```python
from build123d import *

# Parameters (mm, degrees)
SKETCH2_W = 2
SKETCH2_H = 3


with BuildPart() as part:
    # Sweep1: sweep along a path in Sketch1
    with BuildLine(Plane(origin=(0, 0, 0), x_dir=(1, 0, 0), z_dir=(0, 1, 0))) as sweep1_path:
        Line((5.441400564, 4.563847428), (1.294095226, 3.452580312))
        ThreePointArc((1.294095226, 3.452580312), (0, 3.282209443), (-1.294095226, 3.452580312))
        Line((-1.294095226, 3.452580312), (-4.053171996, 4.191872704))
        ThreePointArc((-4.053171996, 4.191872704), (-5.890289303, 3.131212533), (-4.829629131, 1.294095226))
        Line((-4.829629131, 1.294095226), (4.829629131, -1.294095226))
        ThreePointArc((4.829629131, -1.294095226), (5.890289303, -3.131212533), (4.053171996, -4.191872704))
        Line((4.053171996, -4.191872704), (1.294095226, -3.452580312))
        ThreePointArc((1.294095226, -3.452580312), (0, -3.282209443), (-1.294095226, -3.452580312))
        Line((-1.294095226, -3.452580312), (-5.441400564, -4.563847428))
    # Sketch2 → Sweep1 (sweep)
    with BuildSketch(Plane(origin=(-5.441400564, 0, 4.563847428), x_dir=(0.2588190451025149, 0, 0.96592582628907), z_dir=(-0.96592582628907, 0, 0.2588190451025149))):
        Rectangle(SKETCH2_W, SKETCH2_H)
    sweep(path=sweep1_path.line)


solid = part.part
```
Can you work these out from the model? Positions are in its coordinate system, mm. A direction names the side the tool comes from. Round coordinates to 2 decimals unless told otherwise and drop trailing zeros. Loops run counter-clockwise (first coordinate to the right, second up) from the corner with the lowest first, then second, coordinate; pieces in that order, holes last. Notation, with made-up numbers: M 3.25,49 L 29.25,49 A25 cw 29.25,81 Z; hole C -15.75,-10.5 d2. An arc over 180 degrees is marked long. Answer as a JSON object with one key per item and string values. Group by question number.
Q1. Imagine slicing it at B-B, the plane x = 0.25. Please give me the cut outline in (y, z), then the cut area to 3 significant figures.
Q2. Imagine slicing it at C-C, the plane z = 3. Please give me the cut outline in (x, y).
Q3. Please list where these lines run through material, in increasing order: L1, parallel to Z at x = -0.5, y = 0.65; L2, parallel to Z at x = 1.75, y = 1.3; L3, parallel to Z at x = 5, y = -0.35.
Q4. Imagine slicing it at D-D, the plane x = 2. Please give me the cut outline in (y, z), then the cut area to 3 significant figures.
Q5. We'd pull the mould along X, two halves only. Please class faces 6 (the flat face through (0, -1.5, 0)), 7 (the cylindrical face through (0.015, 0.021, 4.282)), 8 (the flat face through (-5.438, -0.021, 4.577)): +X half, -X half, draft (parallel to the pull), parting line (faces both ways), or undercut.
Q6. Imagine slicing it at A-A, the plane y = -0.7. Please give me the cut outline in (x, z), then the cut area to 3 significant figures.
Q7. On a 3-axis mill with a long thin cutter (end or side, diameter ignored), from which of +Z, -Z, +X, -X, +Y, -Y can I reach the whole of each face in a straight line? I mean faces 1 (the flat face through (-2.434, 0.021, -4.793)), 2 (the cylindrical face through (0.022, 0.021, -2.282)), 3 (the flat face through (-3.66, 0.02, 3.05)), 4 (the flat face through (3.598, -0.021, -3.035)), 5 (the flat face through (2.396, -0.021, 4.783)). Say none if no direction works.
Q8. Will these pins go through, and if not, where does the flat tip stop? pin 1 (1.5 mm diameter, centred on x = -1, y = 1, fed in from +Z); pin 2 (1 mm diameter, centred on y = -0.5, z = 0.5, fed in from +X).
Findings:
{
 "1": {"outline": "M -1.5,-4.29 L 1.5,-4.29 L 1.5,-2.29 L -1.5,-2.29 Z; M -1.5,-0.97 L 1.5,-0.97 L 1.5,1.1 L -1.5,1.1 Z; M -1.5,2.29 L 1.5,2.29 L 1.5,4.29 L -1.5,4.29 Z", "area": "18.2 mm2"},
 "2": {"outline": "M -3.47,-1.5 L 3.47,-1.5 L 3.47,1.5 L -3.47,1.5 Z; M 4.87,-1.5 L 6.93,-1.5 L 6.93,1.5 L 4.87,1.5 Z"},
 "3": {"L1": "z = -4.31 to -2.3, -1.17 to 0.9, 2.3 to 4.31", "L2": "z = -4.61 to -2.54, -0.57 to 1.5, 2.54 to 4.61", "L3": "z = -5.48 to -3.41, 0.3 to 5.18"},
 "4": {"outline": "M -1.5,-4.68 L 1.5,-4.68 L 1.5,-2.61 L -1.5,-2.61 Z; M -1.5,-0.5 L 1.5,-0.5 L 1.5,1.57 L -1.5,1.57 Z; M -1.5,2.61 L 1.5,2.61 L 1.5,4.68 L -1.5,4.68 Z", "area": "18.6 mm2"},
 "5": {"face 6": "draft", "face 7": "undercut", "face 8": "-X half"},
 "6": {"outline": "M -5.7,3.6 L -1.55,2.49 A6 ccw 1.55,2.49 L 4.31,3.23 A0.5 cw 4.57,2.26 L -5.09,-0.33 A2.5 ccw -3.79,-5.16 L -1.04,-4.42 A4 cw 1.04,-4.42 L 5.18,-5.53 L 5.7,-3.6 L 1.55,-2.49 A6 ccw -1.55,-2.49 L -4.31,-3.23 A0.5 cw -4.57,-2.26 L 5.09,0.33 A2.5 ccw 3.79,5.16 L 1.04,4.42 A4 cw -1.04,4.42 L -5.18,5.53 Z", "area": "77.9 mm2"},
 "7": {"face 1": "-Z, +Y, -Y", "face 2": "+Y, -Y", "face 3": "-X, +Y, -Y", "face 4": "+X, +Y, -Y", "face 5": "+Z, +Y, -Y"},
 "8": {"pin 1": "stops at z = 4.61", "pin 2": "stops at x = 6.23"}
}
